Build history of the part. All positions in model axes, mm. Face numbers are marked on the shaded views. A direction names the side the tool comes from. Coordinates: 2 decimals unless noted, no trailing zeros. Order: outer loops, then holes, each group sorted by start corner. A loop starts at its lowest first (then second) coordinate and runs counter-clockwise, first axis right, second up. Notation, with made-up numbers: (-3, -36) - (16, -36) arc R28 ccw to (16, -12) - close; hole circle Ø1 at (1.25, -6.75). An arc over 180 degrees is marked (long way). One line per item, written item: value.
from build123d import *

# Parameters (mm, degrees)
SKETCH1_W           = 93
SKETCH1_H           = 100
BOSS_EXTRUDE2_DEPTH = 6.3
SKETCH3_W           = 40
SKETCH3_H           = 100
BOSS_EXTRUDE3_DEPTH = 9.9
SKETCH4_W           = 16.2
SKETCH4_H           = 15
BOSS_EXTRUDE4_DEPTH = 24
SKETCH5_R           = 2
CUT_EXTRUDE1_DEPTH  = 50
SKETCH6_R           = 7.5
CUT_EXTRUDE2_DEPTH  = 50
SKETCH7_R           = 8
CUT_EXTRUDE3_DEPTH  = 50
EXTRUDE_THIN1_START = -5.3
SKETCH7_2_R         = 8
SKETCH7_2_R_2       = 6
EXTRUDE_THIN1_DEPTH = 1
EXTRUDE_THIN2_START = -15.2
SKETCH6_2_R         = 7.5
SKETCH6_2_R_2       = 5.5
EXTRUDE_THIN2_DEPTH = 1
SKETCH8_R           = 1.4
CUT_EXTRUDE4_DEPTH  = 20


with BuildPart() as part:
    # Sketch1 → Boss-Extrude2 (new body)
    with BuildSketch(Plane.XY):
        with Locations((-29.68705036, 14.928057554)):
            Rectangle(SKETCH1_W, SKETCH1_H)
    extrude(amount=BOSS_EXTRUDE2_DEPTH)

    # Sketch3 → Boss-Extrude3 (add)
    with BuildSketch(Plane(origin=(0, 0, 0), x_dir=(-1, 0, 0), z_dir=(0, 0, -1))):
        with Locations((3.18705036, 14.928057554)):
            Rectangle(SKETCH3_W, SKETCH3_H)
    extrude(amount=BOSS_EXTRUDE3_DEPTH)

    # Sketch4 → Boss-Extrude4 (add)
    with BuildSketch(Plane(origin=(16.81294964, 0, 0), x_dir=(0, 0, -1), z_dir=(1, 0, 0))):
        with Locations((1.8, -12.571942446)):
            Rectangle(SKETCH4_W, SKETCH4_H)
    extrude(amount=BOSS_EXTRUDE4_DEPTH)

    # Sketch5 → Cut-Extrude1 (cut)
    with BuildSketch(Plane(origin=(0, -5.071942446, 0), x_dir=(1, 0, 0), z_dir=(0, 1, 0))):
        with Locations(Location((26.81294964, 1.7, 0), (0, 0, 180))):
            Circle(SKETCH5_R)
    extrude(amount=-CUT_EXTRUDE1_DEPTH, mode=Mode.SUBTRACT)

    # Sketch6 → Cut-Extrude2 (cut)
    with BuildSketch(Plane(origin=(0, 0, -9.9), x_dir=(-1, 0, 0), z_dir=(0, 0, -1))):
        with Locations((-1.81294964, -24.571942446)):
            Circle(SKETCH6_R)
    extrude(amount=-CUT_EXTRUDE2_DEPTH, mode=Mode.SUBTRACT)

    # Sketch7 → Cut-Extrude3 (cut)
    with BuildSketch(Plane(origin=(0, 0, 0), x_dir=(-1, 0, 0), z_dir=(0, 0, -1))):
        with Locations((53.18705036, 36.928057554)):
            Circle(SKETCH7_R)
    extrude(amount=-CUT_EXTRUDE3_DEPTH, mode=Mode.SUBTRACT)

    # Sketch7<2> → Extrude-Thin1 (add)
    with BuildSketch(Plane(origin=(0, 0, 0), x_dir=(-1, 0, 0), z_dir=(0, 0, -1)).offset(EXTRUDE_THIN1_START)):
        with Locations((53.18705036, 36.928057554)):
            Circle(SKETCH7_2_R)
        with Locations((53.18705036, 36.928057554)):
            Circle(SKETCH7_2_R_2, mode=Mode.SUBTRACT)
    extrude(amount=-EXTRUDE_THIN1_DEPTH)

    # Sketch6<2> → Extrude-Thin2 (add)
    with BuildSketch(Plane(origin=(0, 0, -9.9), x_dir=(-1, 0, 0), z_dir=(0, 0, -1)).offset(EXTRUDE_THIN2_START)):
        with Locations((-1.81294964, -24.571942446)):
            Circle(SKETCH6_2_R)
        with Locations((-1.81294964, -24.571942446)):
            Circle(SKETCH6_2_R_2, mode=Mode.SUBTRACT)
    extrude(amount=-EXTRUDE_THIN2_DEPTH)

    # Sketch8 → Cut-Extrude4 (cut)
    with BuildSketch(Plane(origin=(0, 64.928057554, 0), x_dir=(1, 0, 0), z_dir=(0, 1, 0))):
        with Locations(Location((-15.68705036, 1.8, 0), (0, 0, 270))):
            Circle(SKETCH8_R)
        with Locations(Location((9.31294964, 1.8, 0), (0, 0, 270))):
            Circle(SKETCH8_R)
    extrude(amount=-CUT_EXTRUDE4_DEPTH, mode=Mode.SUBTRACT)


solid = part.part
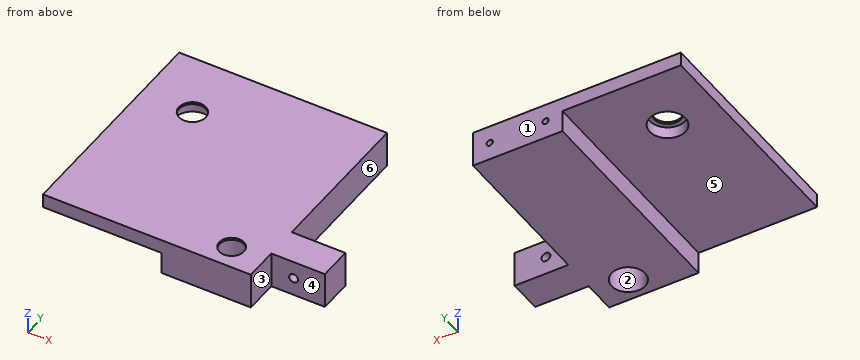
1. Probe line 1 along X through (y, z) = (50.5, -1.8); line 2 along X through (y, z) = (25, -2.25); line 3 along Y through (x, z) = (31, 1.25). List the from-to ranges inside material, lowest first.
Values found:
line 1: x = -23.19 to -17.09, -14.29 to 7.91, 10.71 to 16.81
line 2: x = -23.19 to 16.81
line 3: y = -20.07 to -5.07
2. Flat gauge pins, fed straight in: P1, Ø1.7, axis at x = -15.69, z = -1.8, coming from the +Y side; P2, Ø8, axis at x = -51, y = 36.5, coming from the -Z side; P3, Ø4.5, axis at x = 2.5, y = -21.5, coming from the -Z side; P4, Ø1.5, axis at y = 11.5, z = -0.5, coming from the -X side. Where does each tip first touch, or does it go through?
Values found:
P1: stops at y = 44.93
P2: stops at z = 5.3
P3: passes through
P4: stops at x = -76.19
3. Band-saw the part on D-D, the plane y = 6. Give the cut face in (x, z), and give its area (3 significant figures).
Values found:
outline: (-76.19, 0) - (-23.19, 0) - (-23.19, -9.9) - (16.81, -9.9) - (16.81, 6.3) - (-76.19, 6.3) - close
area: 982 mm2
4. Band-saw the part on C-C, the plane y = 38.5. Give the cut face in (x, z).
Values found:
outline: (-76.19, 0) - (-61.03, 0) - (-61.03, 5.3) - (-58.98, 5.3) - (-58.98, 6.3) - (-76.19, 6.3) - close; (-47.4, 5.3) - (-45.34, 5.3) - (-45.34, 0) - (-23.19, 0) - (-23.19, -9.9) - (16.81, -9.9) - (16.81, 6.3) - (-47.4, 6.3) - close
5. Band-saw the part on A-A, the plane z = -1.7. Give the cut face in (x, y), and give its area (3 significant figures).
Values found:
outline: (-23.19, -35.07) - (16.81, -35.07) - (16.81, -20.07) - (24.81, -20.07) - (24.81, -5.07) - (16.81, -5.07) - (16.81, 64.93) - (10.71, 64.93) - (10.71, 44.93) - (7.92, 44.93) - (7.92, 64.93) - (-14.29, 64.93) - (-14.29, 44.93) - (-17.08, 44.93) - (-17.08, 64.93) - (-23.19, 64.93) - close; (28.81, -20.07) - (40.81, -20.07) - (40.81, -5.07) - (28.81, -5.07) - close; hole circle Ø15 at (1.81, -24.57)
area: 4,010 mm2
6. 3-axis set-ups, long thin cutter, end or side, ignore diameter. For the marked faces 4, 5 and 6: which of +Z, -Z, +X, -X, +Y, -Y reach the whole face in a straight line?
Values found:
face 4: +Z, -Z, +X, -Y
face 5: -Z, -X, +Y, -Y
face 6: +Z, -Z, +X, +Y
7. Two-plate mould, pull along Y, no slides. Class the marked faces 1, 2 and 3: pulls with the +Y half, pulls with the -Y half, needs draft (parallel to the pull), parting line crosses it, or undercut.
Values found:
face 1: pulls with the +Y half
face 2: undercut
face 3: needs draft
8. Band-saw the part on B-B, the plane x = 27. Give the cut face in (y, z).
Values found:
outline: (-20.07, -9.9) - (-5.07, -9.9) - (-5.07, -3.69) - (-20.07, -3.69) - close; (-20.07, 0.29) - (-5.07, 0.29) - (-5.07, 6.3) - (-20.07, 6.3) - close
